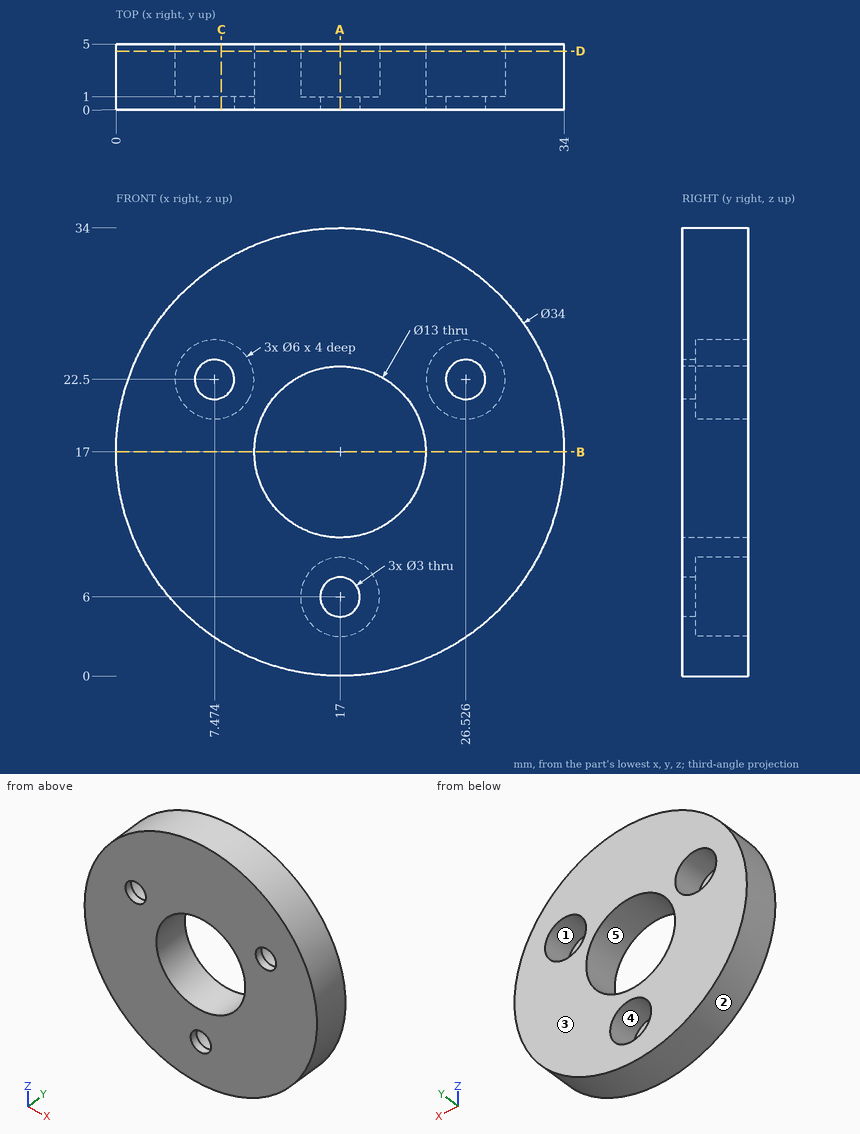
Geometry: see drawing. Coordinates: mm, zero at the bounding-box minimum. A direction names the side the tool comes from. Round coordinates to 2 decimals unless told otherwise and drop trailing zeros. Order: outer loops, then holes, each group sorted by start corner. A loop starts at its lowest first (then second) coordinate and runs counter-clockwise, first axis right, second up. Notation, with made-up numbers: (54.25, 23.25) -> (105.25, 23.25) arc R12 ccw to (105.25, 39.25) -> close; hole circle Ø8 at (35, 17). An arc over 180 degrees is marked (long way). Write each question's results on one line, items separated by ' | '.
Q1. Section query A-A (x = 17). Output: boundary loops of the cut face in (y, z).
Response values:
outline: (0, 0) -> (5, 0) -> (5, 3) -> (1, 3) -> (1, 4.5) -> (0, 4.5) -> close; (0, 7.5) -> (1, 7.5) -> (1, 9) -> (5, 9) -> (5, 10.5) -> (0, 10.5) -> close; (0, 23.5) -> (5, 23.5) -> (5, 34) -> (0, 34) -> close
Q2. Section query D-D (y = 4.45). Output: boundary loops of the cut face in (x, z), and give its area (3 significant figures).
Response values:
outline: circle Ø34 at (17, 17); hole circle Ø6 at (7.47, 22.5); hole circle Ø13 at (17, 17); hole circle Ø6 at (17, 6); hole circle Ø6 at (26.53, 22.5) | area: 690 mm²
Q3. Section query C-C (x = 8). Output: boundary loops of the cut face in (y, z) (1 decimal), and give its area (3 significant figures).
Response values:
outline: (0, 2.6) -> (5, 2.6) -> (5, 19.5) -> (1, 19.5) -> (1, 21.1) -> (0, 21.1) -> close; (0, 23.9) -> (1, 23.9) -> (1, 25.5) -> (5, 25.5) -> (5, 31.4) -> (0, 31.4) -> close | area: 118 mm²
Q4. Section query B-B (z = 17). Output: boundary loops of the cut face in (x, y), and give its area (3 significant figures).
Response values:
outline: (0, 0) -> (10.5, 0) -> (10.5, 5) -> (0, 5) -> close; (23.5, 0) -> (34, 0) -> (34, 5) -> (23.5, 5) -> close | area: 105 mm²
Q5. Ray query, line 1 along Z through (x, y) = (17, 2.55); line 2 along X through (y, z) = (0.3, 22.5) (1 decimal); line 3 along Z through (x, y) = (26, 2.7). Return the intervals inside material, ascending.
Response values:
line 1: 0 to 3, 9 to 10.5, 23.5 to 34 | line 2: 0.9 to 6, 9 to 13.5, 20.5 to 25, 28 to 33.1 | line 3: 2.58 to 19.55, 25.45 to 31.42
Q6. Access query for the marked faces 4 and 5. Directions: +Z, -Z, +X, -X, +Y, -Y. A direction counts if a zero-diameter tool reaches every point of the face in a straight line with its end or side. Return the directions, or none.
Response values:
face 4: +Y | face 5: +Y, -Y
Q7. Pin query (flat end, axial travel): pin 1 Ø3 at (x, y) = (30.5, 1.5) entering from -Z; pin 2 Ø1.5 at (y, z) = (1, 30.5) entering from -X (1 decimal); pin 3 Ø3.5 at (x, z) = (26.53, 22.5) entering from +Y. Return the tip coordinate at first contact, or that it passes through.
Response values:
pin 1: z = 4.96 | pin 2: x = 5.8 | pin 3: y = 1
Q8. Pull-direction query (X, two-part tool) for the marked faces 1, 2 and 3; classes: released by +X, released by -X, zero draft, split by the parting line, or undercut.
Response values:
face 1: undercut | face 2: split by the parting line | face 3: zero draft
